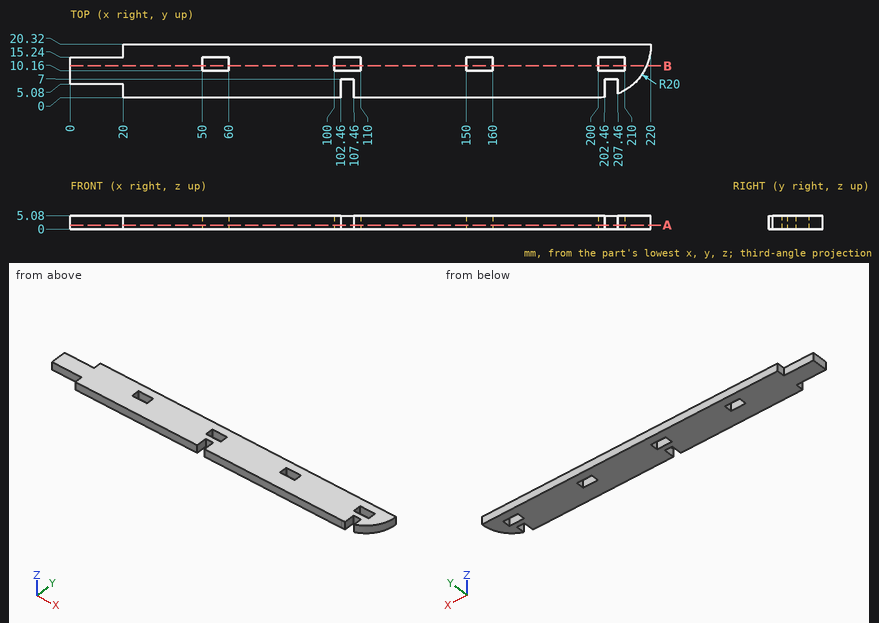
Check sheet for the drawn part. Datum: minimum x, y, z corner. Units: mm. Round coordinates to 2 decimals unless told otherwise and drop trailing zeros. Order: outer loops, then holes, each group sorted by start corner. A loop starts at its lowest first (then second) coordinate and runs counter-clockwise, first axis right, second up.
1. Section check B-B on y = 12. Record the cut outline in (x, z).
Final values:
outline: (0, 0) - (50, 0) - (50, 5.08) - (0, 5.08) - close; (60, 0) - (100, 0) - (100, 5.08) - (60, 5.08) - close; (110, 0) - (150, 0) - (150, 5.08) - (110, 5.08) - close; (160, 0) - (200, 0) - (200, 5.08) - (160, 5.08) - close; (210, 0) - (218.33, 0) - (218.33, 5.08) - (210, 5.08) - close
2. Section check A-A on z = 1.5. State how many separate pieces and enclosed holes the cut face has, then the cut area to 3 significant figures.
Final values:
separate pieces: 1
enclosed holes: 4
area: 3,910 mm2
3. Thickness scan on L1, parallel to X at y = 4.75, z = 2.2; L2, parallel to X at y = 5.5, z = 2.2; L3, parallel to X at y = 10.25, z = 4.25. Record the ranges inside material, lowest first.
Final values:
L1: x = 20 to 102.46, 107.46 to 202.46, 207.46 to 212.94
L2: x = 0 to 102.46, 107.46 to 202.46, 207.46 to 213.77
L3: x = 0 to 50, 60 to 100, 110 to 150, 160 to 200, 210 to 217.46
4. Go/stop test with flat-tipped pins: P1, Ø1.5, axis at y = 13.5, z = 3, coming from the +X side; P2, Ø2.5, axis at x = 12, z = 2, coming from the -Y side; P3, Ø1.5, axis at y = 2.5, z = 1.5, coming from the -X side. Record where each tip stops, or that it passes through.
Final values:
P1: stops at x = 219.16
P2: stops at y = 5.08
P3: stops at x = 20
